Here's how the part is built. I have some questions about the finished solid (model axes, mm). Face numbers are marked on the shaded views. A direction names the side the tool comes from. Round coordinates to 2 decimals unless told otherwise and drop trailing zeros. Order: outer loops, then holes, each group sorted by start corner. A loop starts at its lowest first (then second) coordinate and runs counter-clockwise, first axis right, second up. Notation, with made-up numbers: (69, 87) - (94, 87) arc R22 ccw to (94, 125) - close; hole circle Ø11 at (18, 77). An arc over 180 degrees is marked (long way). One line per item, written item: value.
from build123d import *

# Parameters (mm, degrees)
EXTRUDE_1_DEPTH     = 20
CUT_EXTRUDE_2_DEPTH = 32.272991542


with BuildPart() as part:
    # 草图1 → 凸台-拉伸1 (new body)
    with BuildSketch(Plane.XY):
        with BuildLine():
            Line((6.767949192, 15.722431864), (5.700983566, 13.87439319))
            ThreePointArc((5.700983566, 13.87439319), (3.882285677, 14.488887394), (2, 14.866068747))
            Line((2, 14.866068747), (2, 17))
            Line((2, 17), (-2, 17))
            Line((-2, 17), (-2, 14.866068747))
            ThreePointArc((-2, 14.866068747), (-3.882285677, 14.488887394), (-5.700983566, 13.87439319))
            Line((-5.700983566, 13.87439319), (-6.767949192, 15.722431864))
            Line((-6.767949192, 15.722431864), (-10.232050808, 13.722431864))
            Line((-10.232050808, 13.722431864), (-9.165085181, 11.87439319))
            ThreePointArc((-9.165085181, 11.87439319), (-10.606601718, 10.606601718), (-11.87439319, 9.165085181))
            Line((-11.87439319, 9.165085181), (-13.722431864, 10.232050808))
            Line((-13.722431864, 10.232050808), (-15.722431864, 6.767949192))
            Line((-15.722431864, 6.767949192), (-13.87439319, 5.700983566))
            ThreePointArc((-13.87439319, 5.700983566), (-14.488887394, 3.882285677), (-14.866068747, 2))
            Line((-14.866068747, 2), (-17, 2))
            Line((-17, 2), (-17, -2))
            Line((-17, -2), (-14.866068747, -2))
            ThreePointArc((-14.866068747, -2), (-14.488887394, -3.882285677), (-13.87439319, -5.700983566))
            Line((-13.87439319, -5.700983566), (-15.722431864, -6.767949192))
            Line((-15.722431864, -6.767949192), (-13.722431864, -10.232050808))
            Line((-13.722431864, -10.232050808), (-11.87439319, -9.165085181))
            ThreePointArc((-11.87439319, -9.165085181), (-10.606601718, -10.606601718), (-9.165085181, -11.87439319))
            Line((-9.165085181, -11.87439319), (-10.232050808, -13.722431864))
            Line((-10.232050808, -13.722431864), (-6.767949192, -15.722431864))
            Line((-6.767949192, -15.722431864), (-5.700983566, -13.87439319))
            ThreePointArc((-5.700983566, -13.87439319), (-3.882285677, -14.488887394), (-2, -14.866068747))
            Line((-2, -14.866068747), (-2, -17))
            Line((-2, -17), (2, -17))
            Line((2, -17), (2, -14.866068747))
            ThreePointArc((2, -14.866068747), (3.882285677, -14.488887394), (5.700983566, -13.87439319))
            Line((5.700983566, -13.87439319), (6.767949192, -15.722431864))
            Line((6.767949192, -15.722431864), (10.232050808, -13.722431864))
            Line((10.232050808, -13.722431864), (9.165085181, -11.87439319))
            ThreePointArc((9.165085181, -11.87439319), (10.606601718, -10.606601718), (11.87439319, -9.165085181))
            Line((11.87439319, -9.165085181), (13.722431864, -10.232050808))
            Line((13.722431864, -10.232050808), (15.722431864, -6.767949192))
            Line((15.722431864, -6.767949192), (13.87439319, -5.700983566))
            ThreePointArc((13.87439319, -5.700983566), (14.488887394, -3.882285677), (14.866068747, -2))
            Line((14.866068747, -2), (17, -2))
            Line((17, -2), (17, 2))
            Line((17, 2), (14.866068747, 2))
            ThreePointArc((14.866068747, 2), (14.488887394, 3.882285677), (13.87439319, 5.700983566))
            Line((13.87439319, 5.700983566), (15.722431864, 6.767949192))
            Line((15.722431864, 6.767949192), (13.722431864, 10.232050808))
            Line((13.722431864, 10.232050808), (11.87439319, 9.165085181))
            ThreePointArc((11.87439319, 9.165085181), (10.606601718, 10.606601718), (9.165085181, 11.87439319))
            Line((9.165085181, 11.87439319), (10.232050808, 13.722431864))
            Line((10.232050808, 13.722431864), (6.767949192, 15.722431864))
        make_face()
    extrude(amount=EXTRUDE_1_DEPTH)

    # 草图2 → 切除-拉伸2 (cut, through all)
    with BuildSketch(Plane.XY.offset(20)):
        with BuildLine():
            Line((2.624865364, 11.5), (-2.624865364, 11.5))
            Line((-2.624865364, 11.5), (-2.624865364, 9.64935655))
            ThreePointArc((-2.624865364, 9.64935655), (0, 10), (2.624865364, 9.64935655))
            Line((2.624865364, 9.64935655), (2.624865364, 11.5))
        make_face()
        with BuildLine():
            ThreePointArc((2.624865364, 9.64935655), (0, 10), (-2.624865364, 9.64935655))
            Line((-2.624865364, 9.64935655), (-2.624865364, 8.5))
            Line((-2.624865364, 8.5), (2.624865364, 8.5))
            Line((2.624865364, 8.5), (2.624865364, 9.64935655))
        make_face()
        with BuildLine():
            Line((-2.624865364, 8.5), (-2.624865364, 9.64935655))
            ThreePointArc((-2.624865364, 9.64935655), (-6.072534329, -7.945081927), (10, 0))
            ThreePointArc((10, 0), (7.945081927, 6.072534329), (2.624865364, 9.64935655))
            Line((2.624865364, 9.64935655), (2.624865364, 8.5))
            Line((2.624865364, 8.5), (-2.624865364, 8.5))
        make_face()
    extrude(amount=-CUT_EXTRUDE_2_DEPTH, mode=Mode.SUBTRACT)


solid = part.part
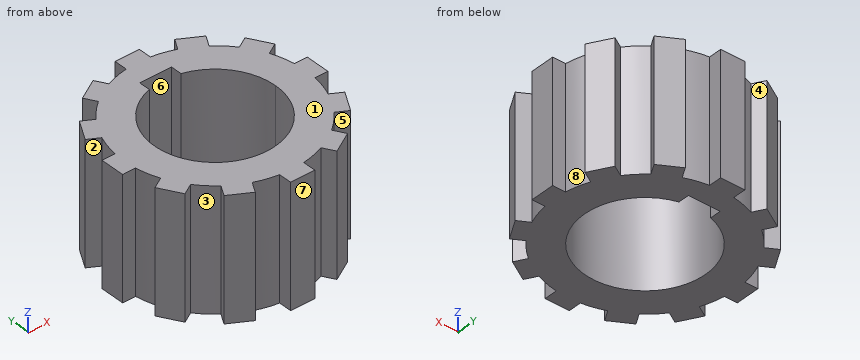
Q1. If I drill on line 1 along Y through (x, z) = (0, 5.75); line 2 along X through (y, z) = (0, 10.5); line 3 along X through (y, z) = (-15, 10), over which ranges is the centre line in solid material (lowest first)?
Results list:
line 1: -17 to -10, 11.5 to 17
line 2: -17 to -10, 10 to 17
line 3: -8.02 to -6.35, -2 to 2, 6.35 to 8.02
Q2. Which directions (+Z, -Z, +X, -X, +Y, -Y) give clear straight access to the entire face, cutting with the end or side of a thin tool? Please do the marked faces 1, 2, 3, 4 and 5.
Results list:
face 1: +Z, +X, -X, +Y, -Y
face 2: +Z, -Z, -X
face 3: +Z, -Z
face 4: +Z, -Z, +Y
face 5: +Z, -Z, -Y
Q3. If we section it at A-A, the plane x = 0: Please give me the cut outline in (y, z).
Results list:
outline: (-17, 0) - (-10, 0) - (-10, 20) - (-17, 20) - close; (11.5, 0) - (17, 0) - (17, 20) - (11.5, 20) - close
Q4. If we section it at C-C, the plane x = -13: Please give me the cut outline in (y, z), then the cut area to 3 significant figures.
Results list:
outline: (-9.81, 0) - (9.81, 0) - (9.81, 20) - (-9.81, 20) - close
area: 393 mm²
Q5. We'd pull the mould along X, two halves only. Please class the marked faces 6, 7 and 8: released by +X, released by -X, zero draft, split by the parting line, or undercut.
Results list:
face 6: undercut
face 7: zero draft
face 8: released by +X
Q6. Will these pins go through, and if not, where does the flat tip stop? pin 1 (6 mm diameter, centred on y = -12, z = 6, fed in from -X); pin 2 (2 mm diameter, centred on y = 12.5, z = 13, fed in from +X); pin 3 (2.5 mm diameter, centred on y = -16.5, z = 14, fed in from -X).
Results list:
pin 1: x = -14.43
pin 2: x = 10.1
pin 3: x = -7.59
Q7. If we section it at B-B, the plane y = 5: Please give me the cut outline in (x, z).
Results list:
outline: (-14.14, 0) - (-8.66, 0) - (-8.66, 20) - (-14.14, 20) - close; (8.66, 0) - (14.14, 0) - (14.14, 20) - (8.66, 20) - close
